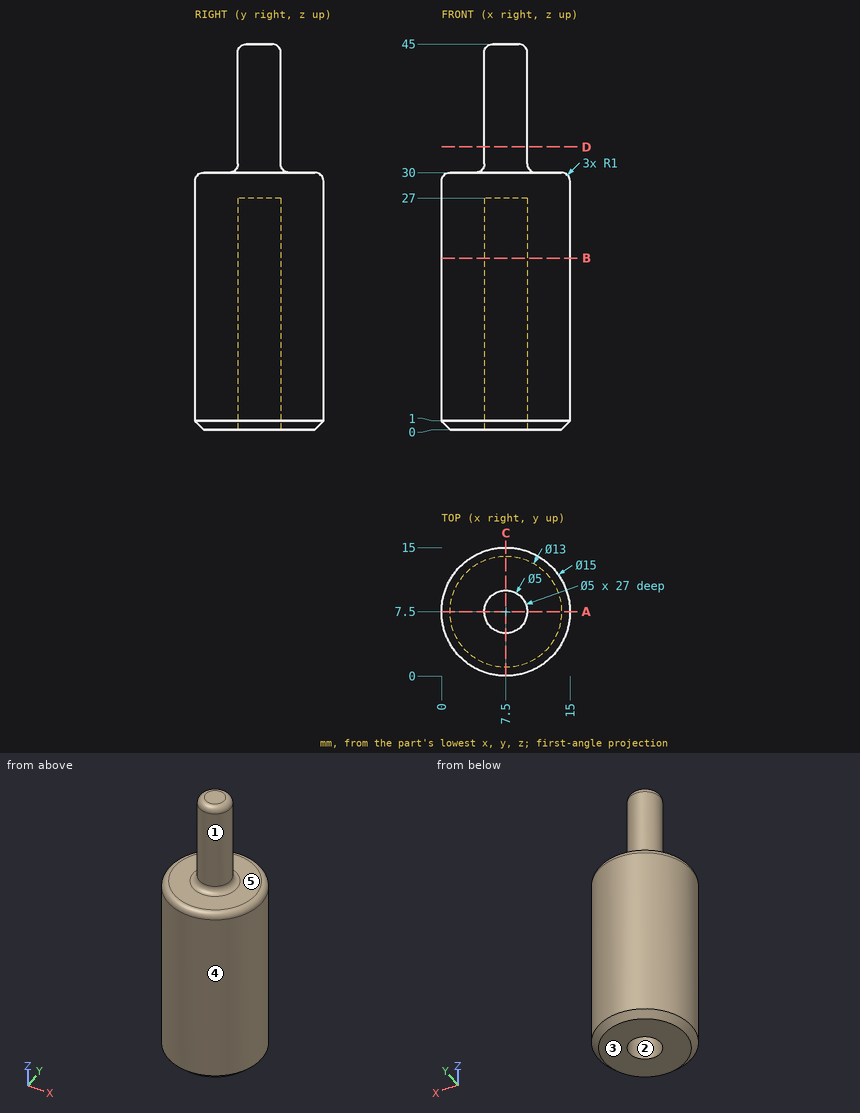
Could you check a few things on this drawing? It's one solid part, dimensions in mm from its lowest x, y, z. A direction names the side the tool comes from. Round coordinates to 2 decimals unless told otherwise and drop trailing zeros. Loops run counter-clockwise (first coordinate to the right, second up) from the corner with the lowest first, then second, coordinate; pieces in that order, holes last. Notation, with made-up numbers: (5.5, -12) -> (37.5, -12) arc R23 cw to (37.5, 5) -> close; hole circle Ø6 at (3.25, 82). An arc over 180 degrees is marked (long way). One line per item, written item: value. Start each with the question number.
1. If I drill on probe 1 along X at (y, z) = (7.5, 9.75); probe 2 along Z at (x, y) = (3.5, 6.25); probe 3 along Z at (x, y) = (8.5, 8.5), over which ranges is the centre line in solid material (lowest first)?
2. If we section it at A-A, the plane y = 7.5: Write out the boundary of the cut face in (x, z), then the cut area to 3 significant figures.
3. For the marked faces 4 and 5, which set-ups out of +Z, -Z, +X, -X, +Y, -Y let a thin tool reach every point of the face, with its end or its side?
4. If we section it at B-B, the plane z = 20: Write out the boundary of the cut face in (x, y).
5. For pin 1 (2 mm diameter, centred on y = 4, z = 16.5, fed in from +X); pin 2 (4 mm diameter, centred on x = 7.5, y = 7.5, fed in from -Z); pin 3 (5 mm diameter, centred on y = 11.5, z = 29.5, fed in from +X), each with a flat end and sliding along its axis, tell me the tip position at first contact or that it passes through.
6. If we section it at D-D, the plane z = 33: Write out the boundary of the cut face in (x, y), then the cut area to 3 significant figures.
7. If we mould it in two halves opening along X, with no side actions, what happens to the marked faces 1, 2 and 3? For each: pulls with the +X half, pulls with the -X half, needs draft (parallel to the pull), parting line crosses it, or undercut.
Calculated:
1. probe 1: x = 0 to 5, 10 to 15
1. probe 2: z = 0 to 30
1. probe 3: z = 27 to 45
2. outline: (0, 1) -> (1, 0) -> (5, 0) -> (5, 27) -> (10, 27) -> (10, 0) -> (14, 0) -> (15, 1) -> (15, 29) arc R1 ccw to (14, 30) -> (11, 30) arc R1 cw to (10, 31) -> (10, 44) arc R1 ccw to (9, 45) -> (6, 45) arc R1 ccw to (5, 44) -> (5, 31) arc R1 cw to (4, 30) -> (1, 30) arc R1 ccw to (0, 29) -> close
2. area: 389 mm²
3. face 4: +Z, -Z
3. face 5: +Z
4. outline: circle Ø15 at (7.5, 7.5); hole circle Ø5 at (7.5, 7.5)
5. pin 1: stops at x = 14.57
5. pin 2: stops at z = 27
5. pin 3: stops at x = 14.84
6. outline: circle Ø5 at (7.5, 7.5)
6. area: 19.6 mm²
7. face 1: parting line crosses it
7. face 2: undercut
7. face 3: needs draft
